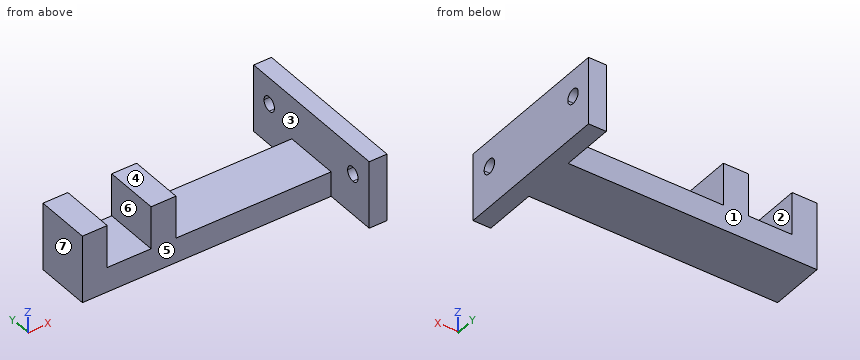
from build123d import *

# Parameters (mm, degrees)
F0_W     = 7
F0_H     = 15.5
F0_W_2   = 12.34
F0_W_3   = 43.66
F0_W_4   = 5
F1_DEPTH = 7
F0_H_2   = 15
F2_DEPTH = 19
F4_DEPTH = 15


with BuildPart() as f1:
    # F0 (on Top) → F1 (new body)
    with BuildSketch(Plane.XY):
        with Locations((-94.8272068564, 0)):
            Rectangle(F0_W, F0_H)
        with Locations((-85.1572068564, 0)):
            Rectangle(F0_W_2, F0_H)
        with Locations((-75.4872068564, 0)):
            Rectangle(F0_W, F0_H)
        with Locations((-50.1572068564, 0)):
            Rectangle(F0_W_3, F0_H)
        with Locations((-25.8272068564, 0)):
            Rectangle(F0_W_4, F0_H)
    extrude(amount=F1_DEPTH)

    # F0 (on Top) → F2 (join)
    with BuildSketch(Plane.XY):
        with Locations((-94.8272068564, 0)):
            Rectangle(F0_W, F0_H)
        with Locations((-75.4872068564, 0)):
            Rectangle(F0_W, F0_H)
        with Locations((-25.8272068564, 0)):
            Rectangle(F0_W_4, F0_H)
        with Locations((-25.8272068564, 15.25)):
            Rectangle(F0_W_4, F0_H_2)
        with Locations((-25.8272068564, -15.25)):
            Rectangle(F0_W_4, F0_H_2)
    extrude(amount=F2_DEPTH)

    # F3 (on face) → F4 (cut)
    with BuildSketch(Plane.YZ.offset(-23.3272068564)):
        with BuildLine():
            ThreePointArc((-14.2406609476, 11.55), (-16.2906609476, 13.6), (-18.3406609476, 11.55))
            Line((-18.3406609476, 11.55), (-14.2406609476, 11.55))
        make_face()
        with BuildLine():
            ThreePointArc((-18.3406609476, 11.55), (-17.740229849, 10.1004310986), (-16.2906609476, 9.5))
            ThreePointArc((-16.2906609476, 9.5), (-14.8410920461, 10.1004310986), (-14.2406609476, 11.55))
            Line((-14.2406609476, 11.55), (-18.3406609476, 11.55))
        make_face()
        with BuildLine():
            ThreePointArc((18.6963237256, 11.55), (16.6463237256, 13.6), (14.5963237256, 11.55))
            Line((14.5963237256, 11.55), (18.6963237256, 11.55))
        make_face()
        with BuildLine():
            ThreePointArc((14.5963237256, 11.55), (15.1967548241, 10.1004310986), (16.6463237256, 9.5))
            ThreePointArc((16.6463237256, 9.5), (18.095892627, 10.1004310986), (18.6963237256, 11.55))
            Line((18.6963237256, 11.55), (14.5963237256, 11.55))
        make_face()
    extrude(amount=-F4_DEPTH, mode=Mode.SUBTRACT)


solid = f1.part
Here's how the part is built. I have some questions about the finished solid (model axes, mm). Face numbers are marked on the shaded views. A direction names the side the tool comes from. Coordinates: 2 decimals unless noted, no trailing zeros. Write each loop counter-clockwise with the first axis right and the second up, starting at its lowest first coordinate (ties: lowest second). Pieces come first, ordered by that corner, then holes.
1) Thinking about a two-plate mould opening in X: for the marked faces 5, 6 and 7, which applies, +X half, -X half, draft (parallel to the pull), parting line (faces both ways), or undercut?
Filled in:
face 5: draft
face 6: undercut
face 7: -X half
2) If we section it at C-C (z = 10.25): List the corners of the cut face in (x, y) for me, plus the area to 3 significant figures.
Filled in:
outline: (-98.33, -7.75) - (-91.33, -7.75) - (-91.33, 7.75) - (-98.33, 7.75) - close; (-78.99, -7.75) - (-71.99, -7.75) - (-71.99, 7.75) - (-78.99, 7.75) - close; (-28.33, -22.75) - (-23.33, -22.75) - (-23.33, -17.88) - (-28.33, -17.88) - close; (-28.33, -14.71) - (-23.33, -14.71) - (-23.33, 15.06) - (-28.33, 15.06) - close; (-28.33, 18.23) - (-23.33, 18.23) - (-23.33, 22.75) - (-28.33, 22.75) - close
area: 413 mm2
3) I'm going to push flat-ended pins straight in: pin 1 (6 mm diameter, centred on x = -37, y = -4.5, fed in from +Z); pin 2 (9.5 mm diameter, centred on x = -62.5, z = 11, fed in from -Y). Where does each tip first touch, or does it pass through?
Filled in:
pin 1: stops at z = 7
pin 2: stops at y = -7.75
4) Which directions (+Z, -Z, +X, -X, +Y, -Y) give clear straight access to the entire face, cutting with the end or side of a thin tool? Please do the marked faces 1, 2, 3 and 4.
Filled in:
face 1: +Z, -Z, -X, +Y
face 2: +Z, +Y, -Y
face 3: +Z
face 4: +Z, +X, -X, +Y, -Y
5) If I drill on line 1 (X direction, y = 1, z = 17.5); line 2 (X direction, y = -12.5, z = 8.25); line 3 (Y direction, x = -76.5, z = 8), over which ranges is the centre line in solid material (lowest first)?
Filled in:
line 1: x = -98.33 to -91.33, -78.99 to -71.99, -28.33 to -23.33
line 2: x = -28.33 to -23.33
line 3: y = -7.75 to 7.75
6) If we section it at A-A (z = 14.75): List the corners of the cut face in (x, y) for me, plus the area to 4 significant figures.
Filled in:
outline: (-98.33, -7.75) - (-91.33, -7.75) - (-91.33, 7.75) - (-98.33, 7.75) - close; (-78.99, -7.75) - (-71.99, -7.75) - (-71.99, 7.75) - (-78.99, 7.75) - close; (-28.33, -22.75) - (-23.33, -22.75) - (-23.33, 22.75) - (-28.33, 22.75) - close
area: 444.5 mm2
7) If we section it at D-D (y = 3.5): List the corners of the cut face in (x, z) for me.
Filled in:
outline: (-98.33, 0) - (-23.33, 0) - (-23.33, 19) - (-28.33, 19) - (-28.33, 7) - (-71.99, 7) - (-71.99, 19) - (-78.99, 19) - (-78.99, 7) - (-91.33, 7) - (-91.33, 19) - (-98.33, 19) - close
8) If we section it at B-B (y = 17.5): List the corners of the cut face in (x, z) for me.
Filled in:
outline: (-28.33, 0) - (-23.33, 0) - (-23.33, 9.69) - (-28.33, 9.69) - close; (-28.33, 13.41) - (-23.33, 13.41) - (-23.33, 19) - (-28.33, 19) - close
